The model under review builds one solid part; all positions refer to its coordinate system, in mm. A direction names the side the tool comes from. Round coordinates to 2 decimals unless told otherwise and drop trailing zeros. Order: outer loops, then holes, each group sorted by start corner. A loop starts at its lowest first (then second) coordinate and runs counter-clockwise, first axis right, second up. Notation, with made-up numbers: (-36, -18) - (-6, -18) arc R24 cw to (-6, 13) - close; hole circle Ø9 at (17.25, 59.5). An arc over 180 degrees is marked (long way). One line per question, with ' | ' between items. Start each with the question number.
Item 1: Tool access review of faces 1 (the face through (15.83, -4.71, 30.27)), 2 (the face through (5.06, -15.83, 7.83)), 3 (the face through (14, -32.4, 15.8)), 4 (the face through (29.38, -29.246, 27.447)): name each direction out of +Z, -Z, +X, -X, +Y, -Y from which nothing blocks a thin tool from reaching the whole face with its end or side.
Item 2: Add section A-A on z = 32. State the section outline as (x, y) points.
Item 3: Draft analysis for pull direction X (two halves, no side actions). For faces 5 (the face through (12.7, -9, 23)), 6 (the face through (25.4, -30, 23)), 7 (the face through (28.68, -5.72, 13.43)), state which applies: +X half, -X half, draft (parallel to the pull), parting line (faces both ways), or undercut.
Item 4: Add section D-D on y = -7. State the section outline as (x, z) points (3 decimals), and give its area (3 significant figures).
Item 5: For L1, parallel to Y at x = 36, z = 11.5; L2, parallel to Y at x = 9, z = 24; L3, parallel to X at y = -22, z = 19, list the stretches that pass through material, from the lowest coordinate up. Write a range as [from, to].
Item 6: Insertion check: pin 1 Ø5.5 at (x, y) = (8.5, -19) entering from +Z (3 decimals); pin 2 Ø3 at (x, y) = (19.5, -6.5) entering from -Z (3 decimals); pin 3 Ø4 at (y, z) = (-13, 21.5) entering from +X. Each pin has a flat end and moves straight along its axis. Give the tip position at first contact, or say it passes through.
Item 7: Add section C-C on z = 23. State how many separate pieces and enclosed holes the cut face has, and give its area (3 significant figures).
from build123d import *

# Parameters (mm, degrees)
F0_W      = 38.1
F0_H      = 38.1
F1_DEPTH  = 38.1
F6_DEPTH  = 38.1
F8_DEPTH  = 38.1
F9_W      = 25.4
F9_H      = 7.62
F10_DEPTH = 38.1


with BuildPart() as f1:
    # F0 (on Front) → F1 (new body)
    with BuildSketch(Plane.XZ):
        with Locations((19.05, 19.05)):
            Rectangle(F0_W, F0_H)
    extrude(amount=F1_DEPTH)

    # F5 (on offset) → F6 (cut)
    with BuildSketch(Plane.YZ.offset(38.1)):
        Polygon((-11.43, 18.901093), (-6.35, 38.1), (-31.75, 38.1), (-26.67, 16.491907), (-21.59, 28.575), (-16.51, 28.575), align=None)
        Polygon((-6.35, 0), (0, 0), (0, 38.1), align=None)
        Polygon((-25.4, 0), (-12.7, 0), (-19.05, 15.875), align=None)
        Polygon((-31.75, 0), (-38.1, 38.1), (-38.1, 0), align=None)
    extrude(amount=-F6_DEPTH, mode=Mode.SUBTRACT)

    # F7 (on offset) → F8 (cut)
    with BuildSketch(Plane.XZ.offset(38.1)):
        Polygon((0, 38.1), (0, 0), (6.35, 38.1), align=None)
        Polygon((11.43, 22.225), (6.35, 0), (31.75, 0), (26.67, 22.225), (21.59, 9.525), (16.51, 9.525), align=None)
        Polygon((31.75, 38.1), (38.1, 0), (38.1, 38.1), align=None)
        Polygon((25.4, 38.1), (12.7, 38.1), (19.05, 22.225), align=None)
    extrude(amount=-F8_DEPTH, mode=Mode.SUBTRACT)

    # F9 (on offset) → F10 (cut)
    with BuildSketch(Plane.XY.offset(38.1)):
        with Locations((25.4, -11.43)):
            Rectangle(F9_W, F9_H)
        with Locations((12.7, -26.67)):
            Rectangle(F9_W, F9_H)
    extrude(amount=-F10_DEPTH, mode=Mode.SUBTRACT)


solid = f1.part
Determined:
1) face 1: +Z, +Y, -Y | face 2: -Z, +X, -X | face 3: -Z, +Y, -Y | face 4: +Z, +X, -X
2) outline: (5.33, -37.08) - (15.14, -37.08) - (15.14, -30.48) - (5.33, -30.48) - close; (5.33, -7.96) - (12.7, -7.96) - (12.7, -7.62) - (15.14, -7.62) - (15.14, -1.02) - (5.33, -1.02) - close; (22.96, -37.08) - (32.77, -37.08) - (32.77, -30.32) - (25.4, -30.32) - (25.4, -30.48) - (22.96, -30.48) - close; (22.96, -7.62) - (32.77, -7.62) - (32.77, -1.02) - (22.96, -1.02) - close
3) face 5: +X half | face 6: -X half | face 7: undercut
4) outline: (0, 0) - (6.35, 0) - (11.43, 22.225) - (16.51, 9.525) - (21.59, 9.525) - (26.67, 22.225) - (31.75, 0) - (38.1, 0) - (32.159, 35.643) - (24.417, 35.643) - (19.05, 22.225) - (13.683, 35.643) - (5.941, 35.643) - close | area: 752 mm2
5) L1: [-33.67, -20.8], [-17.3, -15.24], [-7.62, -4.43] | L2: [-35.75, -30.48], [-22.86, -14.11], [-10.08, -2.35] | L3: [3.17, 10.69], [12.72, 25.38], [27.41, 34.93]
6) pin 1: z = 28.575 | pin 2: z = 9.525 | pin 3: x = 12.7
7) separate pieces: 6 | enclosed holes: 0 | area: 600 mm2
